Part model, mm, in its own coordinate system. Face numbers are marked on the shaded views. A direction names the side the tool comes from. Round coordinates to 2 decimals unless told otherwise and drop trailing zeros. Loops run counter-clockwise (first coordinate to the right, second up) from the corner with the lowest first, then second, coordinate; pieces in that order, holes last. Notation, with made-up numbers: (27.25, -34.5) -> (39.25, -34.5) arc R21 ccw to (39.25, -15.5) -> close; hole circle Ø3 at (-5.75, 56.5). An arc over 180 degrees is marked (long way). Answer as CSV lines item,"result".
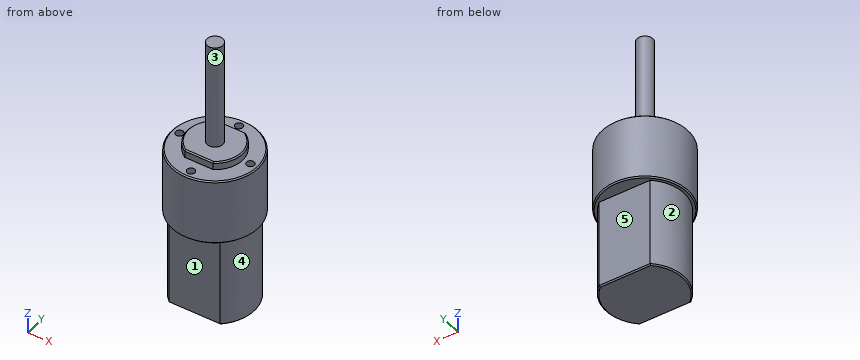
from build123d import *

# Parameters (mm, degrees)
CUT_EXTRUDE1_DEPTH = 23
SKETCH3_R          = 1
CUT_EXTRUDE2_DEPTH = 10
CUT_EXTRUDE3_START = -2
CUT_EXTRUDE3_DEPTH = 2
CHAMFER1_SIZE      = 0.3


with BuildPart() as part:
    # Sketch1 → Revolve1 (revolve)
    with BuildSketch(Plane(origin=(0, 0, 0), x_dir=(1, 0, 0), z_dir=(0, 1, 0)), mode=Mode.PRIVATE) as revolve1_sk:
        Polygon((-2, -29), (-2, -2), (-7, -2), (-7, 0), (-11, 0), (-11, 16.9), (-10, 16.9), (-10, 39.9), (0, 39.9), (0, -29), align=None)
    revolve(revolve1_sk.sketch.rotate(Axis((0, 0, -0.287466161), (0, 0, -1)), 180), axis=Axis((0, 0, -0.287466161), (0, 0, -1)))

    # Sketch2 → Cut-Extrude1 (cut)
    with BuildSketch(Plane(origin=(0, 0, -39.9), x_dir=(-1, 0, 0), z_dir=(0, 0, -1))):
        with BuildLine():
            ThreePointArc((6.469882147, 7.625), (0, 10), (-6.469882147, 7.625))
            Line((-6.469882147, 7.625), (6.469882147, 7.625))
        make_face()
        with BuildLine():
            Line((6.469882147, -7.625), (-6.469882147, -7.625))
            ThreePointArc((-6.469882147, -7.625), (0, -10), (6.469882147, -7.625))
        make_face()
    extrude(amount=-CUT_EXTRUDE1_DEPTH, mode=Mode.SUBTRACT)

    # Sketch3 → Cut-Extrude2 (cut)
    with BuildSketch(Plane.XY):
        with Locations((0, 9)):
            Circle(SKETCH3_R)
        with Locations((9, 0)):
            Circle(SKETCH3_R)
        with Locations((0, -9)):
            Circle(SKETCH3_R)
        with Locations((-9, 0)):
            Circle(SKETCH3_R)
    extrude(amount=-CUT_EXTRUDE2_DEPTH, mode=Mode.SUBTRACT)

    # Sketch4 → Cut-Extrude3 (cut)
    with BuildSketch(Plane.XY.offset(2).offset(CUT_EXTRUDE3_START)):
        with BuildLine():
            ThreePointArc((3.605551275, 6), (0, 7), (-3.605551275, 6))
            Line((-3.605551275, 6), (3.605551275, 6))
        make_face()
        with BuildLine():
            Line((3.605551275, -6), (-3.605551275, -6))
            ThreePointArc((-3.605551275, -6), (0, -7), (3.605551275, -6))
        make_face()
    extrude(amount=CUT_EXTRUDE3_DEPTH, mode=Mode.SUBTRACT)

    # Chamfer1
    chamfer1_edges = [part.edges().sort_by_distance(p)[0] for p in [
        (-11, 0, 0),
        (-10, 0, -39.9),
        (10, 0, -39.9),
        (0, 7.625, -39.9),
        (0, -7.625, -39.9),
        (-7, 0, 2),
        (7, 0, 2),
        (0, 6, 2),
        (0, -6, 2),
        (-11, 0, -16.9),
    ]]
    chamfer(chamfer1_edges, length=CHAMFER1_SIZE)


solid = part.part
Q1. Which spindle directions (+Z, -Z, +X, -X, +Y, -Y) get a long thin tool onto all of the face, cutting with end or side? Do the marked faces 1, 2, 3, 4 and 5. Say none if no direction does.
Geometry results:
face 1,"-Z, +X, -X, -Y"
face 2,"-Z, -X"
face 3,"+Z"
face 4,"-Z, +X"
face 5,"-Z, +X, -X, +Y"
Q2. Drop flat-ended pins along their axis: P1, Ø10, axis at y = -3.5, z = 14.5, coming from the +X side; P2, Ø1.5, axis at y = 5, z = -11, coming from the +X side; P3, Ø0.8, axis at x = 1, z = 1, coming from the +Y side. Give the stop position or say it passes through.
Geometry results:
P1,"x = 2"
P2,"x = 10.15"
P3,"y = 6"
Q3. Saw through at D-D, the plane z = -26.5. Write the cut outline in (x, y) (3 decimals), then the cut area to 3 significant figures.
Geometry results:
outline,"(-6.47, -7.625) -> (6.47, -7.625) arc R10 ccw to (6.47, 7.625) -> (-6.47, 7.625) arc R10 ccw to start"
area,"272 mm2"
Q4. Saw through at B-B, the plane z = -8. Write the cut outline in (x, y).
Geometry results:
outline,"circle Ø22 at (0, 0); hole circle Ø2 at (-9, 0); hole circle Ø2 at (0, -9); hole circle Ø2 at (0, 9); hole circle Ø2 at (9, 0)"
Q5. Drill centre lines: line 1 along Y through (x, z) = (0, -2.5); line 2 along Z through (x, y) = (5, -4); line 3 along Z through (x, y) = (6.5, -8.25). Where is each one in solid material? Low to high.
Geometry results:
line 1,"-11 to -10, -8 to 8, 10 to 11"
line 2,"-39.9 to 2"
line 3,"-16.9 to 0"
